from build123d import *
from build123d.topology import SkipClean

# Parameters (mm, degrees)
SKETCH1_R           = 40
SKETCH1_R_2         = 12.5
BOSS_EXTRUDE1_DEPTH = 6
SKETCH3_R           = 20
SKETCH3_R_2         = 12.5
BOSS_EXTRUDE2_DEPTH = 30
SKETCH4_R           = 20
SKETCH4_R_2         = 16.25
BOSS_EXTRUDE3_DEPTH = 12
BOSS_EXTRUDE4_DEPTH = 42
SKETCH6_R           = 17.6
CUT_EXTRUDE2_DEPTH  = 3
BOSS_EXTRUDE5_START = -6
SKETCH7_R           = 40
SKETCH7_R_2         = 20
BOSS_EXTRUDE5_DEPTH = 6
CUT_EXTRUDE1_REACH  = 76.189
SKETCH2_R           = 4


with BuildPart() as part:
    # Sketch1 → Boss-Extrude1 (new body)
    with BuildSketch(Plane(origin=(0, 0, 0), x_dir=(1, 0, 0), z_dir=(0, 1, 0))):
        with Locations(Location((0, 0, 0), (0, 0, 270))):
            Circle(SKETCH1_R)
        with Locations(Location((0, 0, 0), (0, 0, 270))):
            Circle(SKETCH1_R_2, mode=Mode.SUBTRACT)
    extrude(amount=BOSS_EXTRUDE1_DEPTH)

    # Sketch3 → Boss-Extrude2 (add)
    with BuildSketch(Plane(origin=(0, 6, 0), x_dir=(1, 0, 0), z_dir=(0, 1, 0))):
        with Locations(Location((0, 0, 0), (0, 0, 270))):
            Circle(SKETCH3_R)
        with Locations(Location((0, 0, 0), (0, 0, 270))):
            Circle(SKETCH3_R_2, mode=Mode.SUBTRACT)
    extrude(amount=BOSS_EXTRUDE2_DEPTH)

    # Sketch4 → Boss-Extrude3 (add)
    with BuildSketch(Plane(origin=(0, 36, 0), x_dir=(1, 0, 0), z_dir=(0, 1, 0))):
        with Locations(Location((0, 0, 0), (0, 0, 270))):
            Circle(SKETCH4_R)
        with Locations(Location((0, 0, 0), (0, 0, 270))):
            Circle(SKETCH4_R_2, mode=Mode.SUBTRACT)
    extrude(amount=BOSS_EXTRUDE3_DEPTH)

    # Sketch5 → Boss-Extrude4 (add)
    with SkipClean():  # the faces are left unmerged after this step: merging them gives an invalid solid
        with BuildSketch(Plane(origin=(0, 6, 0), x_dir=(1, 0, 0), z_dir=(0, 1, 0))):
            with BuildLine():
                Line((-16.684833585, -11.027979336), (-30.970921684, -25.314067434))
                ThreePointArc((-30.970921684, -25.314067434), (-28.284271247, -28.284271247), (-25.314067434, -30.970921684))
                Line((-25.314067434, -30.970921684), (-11.027979336, -16.684833585))
                ThreePointArc((-11.027979336, -16.684833585), (-14.142135624, -14.142135624), (-16.684833585, -11.027979336))
            make_face()
            with BuildLine():
                Line((-16.684833585, 11.027979336), (-30.970921684, 25.314067434))
                ThreePointArc((-30.970921684, 25.314067434), (-28.284271247, 28.284271247), (-25.314067434, 30.970921684))
                Line((-25.314067434, 30.970921684), (-11.027979336, 16.684833585))
                ThreePointArc((-11.027979336, 16.684833585), (-14.142135624, 14.142135624), (-16.684833585, 11.027979336))
            make_face()
            with BuildLine():
                Line((11.027979336, 16.684833585), (25.314067434, 30.970921684))
                ThreePointArc((25.314067434, 30.970921684), (28.284271247, 28.284271247), (30.970921684, 25.314067434))
                Line((30.970921684, 25.314067434), (16.684833585, 11.027979336))
                ThreePointArc((16.684833585, 11.027979336), (14.142135624, 14.142135624), (11.027979336, 16.684833585))
            make_face()
            with BuildLine():
                Line((16.684833585, -11.027979336), (30.970921684, -25.314067434))
                ThreePointArc((30.970921684, -25.314067434), (28.284271247, -28.284271247), (25.314067434, -30.970921684))
                Line((25.314067434, -30.970921684), (11.027979336, -16.684833585))
                ThreePointArc((11.027979336, -16.684833585), (14.142135624, -14.142135624), (16.684833585, -11.027979336))
            make_face()
        extrude(amount=BOSS_EXTRUDE4_DEPTH)

    # Sketch6 → Cut-Extrude2 (cut)
    with SkipClean():  # the faces are left unmerged after this step: merging them gives an invalid solid
        with BuildSketch(Plane(origin=(0, 48, 0), x_dir=(1, 0, 0), z_dir=(0, 1, 0))):
            with Locations(Location((0, 0, 0), (0, 0, 270))):
                Circle(SKETCH6_R)
        extrude(amount=-CUT_EXTRUDE2_DEPTH, mode=Mode.SUBTRACT)

    # Sketch7 → Boss-Extrude5 (add)
    with SkipClean():  # the faces are left unmerged after this step: merging them gives an invalid solid
        with BuildSketch(Plane(origin=(0, 48, 0), x_dir=(1, 0, 0), z_dir=(0, 1, 0)).offset(BOSS_EXTRUDE5_START)):
            with Locations(Location((0, 0, 0), (0, 0, 270))):
                Circle(SKETCH7_R)
            Circle(SKETCH7_R_2, mode=Mode.SUBTRACT)
        extrude(amount=BOSS_EXTRUDE5_DEPTH)

    # Cut-Extrude1: up to this face of the body (flat: up to its plane)
    cut_extrude1_end = Plane(part.part.faces().sort_by_distance((0, 48, 29.129034722))[0])
    # Sketch2 → Cut-Extrude1 (cut, up to the picked face)
    with BuildSketch(Plane(origin=(0, 0, 0), x_dir=(1, 0, 0), z_dir=(0, 1, 0)), mode=Mode.PRIVATE) as cut_extrude1_sk1:
        with Locations(Location((0, 30, 0), (0, 0, 270))):
            Circle(SKETCH2_R)
    cut_extrude1_tool1 = split(extrude(cut_extrude1_sk1.sketch, amount=CUT_EXTRUDE1_REACH, mode=Mode.PRIVATE), bisect_by=cut_extrude1_end, keep=Keep.BOTH, mode=Mode.PRIVATE)
    # Sketch2 → Cut-Extrude1 (cut, up to the picked face)
    with BuildSketch(Plane(origin=(0, 0, 0), x_dir=(1, 0, 0), z_dir=(0, 1, 0)), mode=Mode.PRIVATE) as cut_extrude1_sk2:
        with Locations(Location((30, 0, 0), (0, 0, 270))):
            Circle(SKETCH2_R)
    cut_extrude1_tool2 = split(extrude(cut_extrude1_sk2.sketch, amount=CUT_EXTRUDE1_REACH, mode=Mode.PRIVATE), bisect_by=cut_extrude1_end, keep=Keep.BOTH, mode=Mode.PRIVATE)
    # Sketch2 → Cut-Extrude1 (cut, up to the picked face)
    with BuildSketch(Plane(origin=(0, 0, 0), x_dir=(1, 0, 0), z_dir=(0, 1, 0)), mode=Mode.PRIVATE) as cut_extrude1_sk3:
        with Locations(Location((0, -30, 0), (0, 0, 270))):
            Circle(SKETCH2_R)
    cut_extrude1_tool3 = split(extrude(cut_extrude1_sk3.sketch, amount=CUT_EXTRUDE1_REACH, mode=Mode.PRIVATE), bisect_by=cut_extrude1_end, keep=Keep.BOTH, mode=Mode.PRIVATE)
    # Sketch2 → Cut-Extrude1 (cut, up to the picked face)
    with BuildSketch(Plane(origin=(0, 0, 0), x_dir=(1, 0, 0), z_dir=(0, 1, 0)), mode=Mode.PRIVATE) as cut_extrude1_sk4:
        with Locations(Location((-30, 0, 0), (0, 0, 270))):
            Circle(SKETCH2_R)
    cut_extrude1_tool4 = split(extrude(cut_extrude1_sk4.sketch, amount=CUT_EXTRUDE1_REACH, mode=Mode.PRIVATE), bisect_by=cut_extrude1_end, keep=Keep.BOTH, mode=Mode.PRIVATE)
    add(cut_extrude1_tool1.solids().sort_by(Axis((0, 0, -30), (0, 1, 0)))[0], mode=Mode.SUBTRACT)
    add(cut_extrude1_tool2.solids().sort_by(Axis((30, 0, 0), (0, 1, 0)))[0], mode=Mode.SUBTRACT)
    add(cut_extrude1_tool3.solids().sort_by(Axis((0, 0, 30), (0, 1, 0)))[0], mode=Mode.SUBTRACT)
    add(cut_extrude1_tool4.solids().sort_by(Axis((-30, 0, 0), (0, 1, 0)))[0], mode=Mode.SUBTRACT)


solid = part.part
Could you check a few things on this model? Use its own coordinates, in mm. A direction names the side the tool comes from. Give positions to 0.01 mm unless a question says otherwise; leave off trailing zeros. Write each loop counter-clockwise with the first axis right and the second up, starting at its lowest first coordinate (ties: lowest second). Pieces come first, ordered by that corner, then holes. Notation, with made-up numbers: (-26.5, 64) - (-19.5, 64) arc R20 ccw to (-19.5, 93) - close; hole circle Ø6 at (35.25, 37.25). An arc over 180 degrees is marked (long way). Use CSV: the item, a comma, the result in double quotes. Start each with the question number.
Item 1: I want a section at C-C, the plane x = 0. Give the number of separate pieces and of enclosed holes in the cut face, then the cut area to 3 significant figures.
Item 2: I want a section at D-D, the plane x = 21.5. Please give me the cut outline in (y, z).
Item 3: I'm going to push flat-ended pins straight in: pin 1 (8 mm diameter, centred on y = 10, z = 28.5, fed in from -X); pin 2 (4 mm diameter, centred on y = 20, z = 10, fed in from +X); pin 3 (15 mm diameter, centred on x = 0, z = 0, fed in from +Y); pin 4 (1.5 mm diameter, centred on x = -13.5, y = 21, fed in from +Z). Where does each tip first touch, or does it pass through?
Item 4: I want a section at B-B, the plane z = 9.5. Please give me the cut outline in (x, y), then the cut area to 3 significant figures.
Item 5: If I drill on line 1 along X through (y, z) = (3.4, 0); line 2 along Y through (x, z) = (-16, 25); line 3 along Z through (x, y) = (-9.5, 3), over which ranges is the centre line in solid material (lowest first)?
Item 6: I want a section at A-A, the plane y = 23.5. Please give me the cut outline in (x, z).
Item 7: For faces 4 (the face through (-10, 36, 8)), 5 (the face through (-5, 42, -29)), 6 (the face through (29, 42, 5)), which set-ups out of +Z, -Z, +X, -X, +Y, -Y let a thin tool reach every point of the face, with its end or its side?
Item 8: If we mould it in two halves opening along X, with no side actions, what happens to faces 1 (the face through (-23.728, 23.748, -18.071)), 2 (the face through (-8, 48, 17)), 3 (the face through (-16, 45, 5))? For each: pulls with the +X half, pulls with the -X half, needs draft (parallel to the pull), parting line crosses it, or undercut.
Findings:
1,separate pieces,"6"
1,enclosed holes,"0"
1,area,"910 mm2"
2,outline,"(0, -33.73) - (6, -33.73) - (6, -27.16) - (42, -27.16) - (42, -33.73) - (48, -33.73) - (48, 33.73) - (42, 33.73) - (42, 27.16) - (6, 27.16) - (6, 33.73) - (0, 33.73) - close; hole (6, -15.84) - (42, -15.84) - (42, 15.84) - (6, 15.84) - close"
3,pin 1,"stops at x = -30.97"
3,pin 2,"stops at x = 18.33"
3,pin 3,"passes through"
3,pin 4,"stops at z = 19.91"
4,outline,"(-38.86, 0) - (-8.12, 0) - (-8.12, 36) - (-13.18, 36) - (-13.18, 45) - (-14.82, 45) - (-14.82, 48) - (-38.86, 48) - (-38.86, 42) - (-17.6, 42) - (-17.6, 6) - (-38.86, 6) - close; (8.12, 0) - (38.86, 0) - (38.86, 6) - (17.6, 6) - (17.6, 42) - (38.86, 42) - (38.86, 48) - (14.82, 48) - (14.82, 45) - (13.18, 45) - (13.18, 36) - (8.12, 36) - close"
4,area,"1,290 mm2"
5,line 1,"x = -40 to -34, -26 to -12.5, 12.5 to 26, 34 to 40"
5,line 2,"y = 0 to 6, 42 to 48"
5,line 3,"z = -38.86 to -8.12, 8.12 to 38.86"
6,outline,"(-30.97, -25.31) arc R40 ccw to (-25.31, -30.97) - (-11.03, -16.68) arc R20 ccw to (11.03, -16.68) - (25.31, -30.97) arc R40 ccw to (30.97, -25.31) - (16.68, -11.03) arc R20 ccw to (16.68, 11.03) - (30.97, 25.31) arc R40 ccw to (25.31, 30.97) - (11.03, 16.68) arc R20 ccw to (-11.03, 16.68) - (-25.31, 30.97) arc R40 ccw to (-30.97, 25.31) - (-16.68, 11.03) arc R20 ccw to (-16.68, -11.03) - close; hole circle Ø25 at (0, 0)"
7,face 4,"+Y"
7,face 5,"-Z"
7,face 6,"+X"
8,face 1,"pulls with the -X half"
8,face 2,"needs draft"
8,face 3,"undercut"
